Source: CAD feature listing. Evaluate the final solid. Frame: model axes, mm. Face numbers are marked on the shaded views. A direction names the side the tool comes from. Give positions to 0.01 mm unless a question says otherwise; leave off trailing zeros. Loops run counter-clockwise (first coordinate to the right, second up) from the corner with the lowest first, then second, coordinate; pieces in that order, holes last. Notation, with made-up numbers: M 23.5,26 L 32.5,26 A25 cw 32.5,50 Z; hole C 39,9 d7. An arc over 180 degrees is marked long. Put each result on its own line as item: value. Start each with the question number.
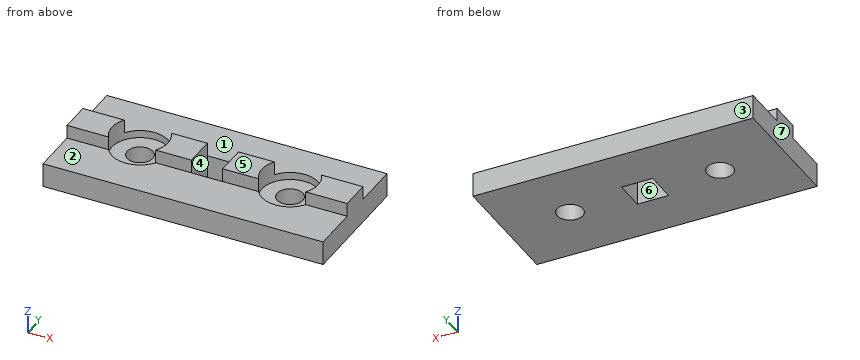
Autodesk Inventor part; units mm, degrees
ref_plane "i1_XY" through (-19.05, 0, -1.905) normal (0, 0, 1) x (1, 0, 0)
ref_plane "i1_YZ" through (-19.05, 0, -1.905) normal (1, 0, 0) x (0, 1, 0)
ref_plane "i1_ZX" through (-19.05, 0, -1.905) normal (0, 1, 0) x (0, 0, 1)
sketch "Sketch_1" plane through (0, 0, 0) normal (1, 0, 0) x (0, 1, 0)
  line L0 (3.9243, 3.429) -> (-3.9243, 3.429)
  line L1 (-3.9243, 3.429) -> (-3.9243, 0)
  line L2 (-3.9243, 0) -> (-15.875, 0)
  line L3 (-15.875, 0) -> (-15.875, -6.096)
  line L4 (-15.875, -6.096) -> (15.875, -6.096)
  line L5 (15.875, -6.096) -> (15.875, 0)
  line L6 (15.875, 0) -> (3.9243, 0)
  line L7 (3.9243, 0) -> (3.9243, 3.429)
extrude "Extrusion1" add sketch "Sketch_1" along normal mid plane 71.12
sketch "Sketch2" plane through (-35.56, 3.9243, 3.429) normal (0, 0, 1) x (1, 0, 0)
  point P0 (16.51, -3.9243)
hole "Drilling 1" at (-19.05, 0, 3.429) direction (0, 0, -1) diameter 6.5278 depth 9.525 counterbore diameter 14.2748 counterbore depth 5.334
sketch "Sketch3" plane through (35.56, -3.9243, 3.429) normal (0, 0, 1) x (1, 0, 0)
  point P0 (-16.51, 3.9243)
hole "Drilling 2" at (19.05, 0, 3.429) direction (0, 0, -1) diameter 6.5278 depth 9.525 counterbore diameter 14.2748 counterbore depth 5.334
sketch "Sketch_4" plane through (0, 0, 0) normal (0, 0, 1) x (1, 0, 0)
  line L0 (-3.9624, -3.9624) -> (3.9624, -3.9624)
  line L1 (3.9624, -3.9624) -> (3.9624, 3.9624)
  line L2 (3.9624, 3.9624) -> (-3.9624, 3.9624)
  line L3 (-3.9624, 3.9624) -> (-3.9624, -3.9624)
extrude "Extrusion2" cut sketch "Sketch_4" along normal mid plane 15.24
ref_plane "i1_XY" through (-19.05, 0, -1.905) normal (0, 0, 1) x (1, 0, 0)
ref_plane "i1_YZ" through (-19.05, 0, -1.905) normal (1, 0, 0) x (0, 1, 0)
ref_plane "i1_ZX" through (-19.05, 0, -1.905) normal (0, 1, 0) x (0, 0, 1)
ref_plane "i2_XY" through (19.05, 0, -1.905) normal (0, 0, 1) x (1, 0, 0)
ref_plane "i2_YZ" through (19.05, 0, -1.905) normal (1, 0, 0) x (0, 1, 0)
ref_plane "i2_ZX" through (19.05, 0, -1.905) normal (0, 1, 0) x (0, 0, 1)
ref_plane "pad_XY" through (-19.05, 0, -6.096) normal (0, 0, 1) x (1, 0, 0)
ref_plane "pad_YZ" through (-19.05, 0, -6.096) normal (1, 0, 0) x (0, 1, 0)
ref_plane "pad_ZX" through (-19.05, 0, -6.096) normal (0, 1, 0) x (0, 0, 1)
properties part number "6596_b"
1. Contact query for flat-ended pins moving along their axis: pin 1 (11.5 mm diameter, centred on x = -19.05, y = 0, fed in from +Z) (3 decimals); pin 2 (2.5 mm diameter, centred on x = 8, z = 2, fed in from -Y); pin 3 (2.5 mm diameter, centred on x = 10, z = 2, fed in from +Y). Output: stop coordinate, or through.
2. Section D-D, the plane z = -5. Output: boundary loops of the cut face in (x, y) (3 decimals).
3. Section C-C, the plane z = 1.5. Output: boundary loops of the cut face in (x, y).
4. Section B-B, the plane x = 2.5. Output: boundary loops of the cut face in (y, z) (3 decimals).
5. Set-up query: the marked faces 1, 2 and 3. Return all of +Z, -Z, +X, -X, +Y, -Y with unobstructed straight access to the full face (end or side cutting, diameter ignored); none if empty.
6. Ray query, line 1 (X direction, y = 0, z = -3.8); line 2 (X direction, y = 0, z = 1.5); line 3 (Y direction, x = -19.05, z = -4.25) (3 decimals). Return the intervals inside material, ascending.
7. Pull-direction query (X, two-part tool) for the marked faces 4, 5, 6 and 7; classes: released by +X, released by -X, zero draft, split by the parting line, or undercut.
8. Section A-A, the plane y = 0. Output: boundary loops of the cut face in (x, z) (3 decimals).
Results found:
1. pin 1: z = -1.905
1. pin 2: y = -3.92
1. pin 3: y = 3.92
2. outline: M -35.56,-15.875 L 35.56,-15.875 L 35.56,15.875 L -35.56,15.875 Z; hole C -19.05,0 d6.528; hole M -3.962,-3.962 L 3.962,-3.962 L 3.962,3.962 L -3.962,3.962 Z; hole C 19.05,0 d6.528
3. outline: M -35.56,-3.92 L -25.01,-3.92 A7.14 cw -25.01,3.92 L -35.56,3.92 Z; M -13.09,-3.92 L -3.96,-3.92 L -3.96,3.92 L -13.09,3.92 A7.14 cw Z; M 3.96,-3.92 L 13.09,-3.92 A7.14 cw 13.09,3.92 L 3.96,3.92 Z; M 25.01,-3.92 L 35.56,-3.92 L 35.56,3.92 L 25.01,3.92 A7.14 cw Z
4. outline: M -15.875,-6.096 L -3.962,-6.096 L -3.962,0 L -15.875,0 Z; M 3.962,-6.096 L 15.875,-6.096 L 15.875,0 L 3.962,0 Z
5. face 1: +Z, +X, -X, +Y
5. face 2: +Z, +X, -X, -Y
5. face 3: +Z, -Z, +X, -X, +Y
6. line 1: -35.56 to -22.31, -15.79 to -3.96, 3.96 to 15.79, 22.31 to 35.56
6. line 2: -35.56 to -26.19, -11.91 to -3.96, 3.96 to 11.91, 26.19 to 35.56
6. line 3: -15.875 to -3.264, 3.264 to 15.875
7. face 4: undercut
7. face 5: zero draft
7. face 6: undercut
7. face 7: released by -X
8. outline: M -35.56,-6.096 L -22.314,-6.096 L -22.314,-1.905 L -26.187,-1.905 L -26.187,3.429 L -35.56,3.429 Z; M -15.786,-6.096 L -3.962,-6.096 L -3.962,3.429 L -11.913,3.429 L -11.913,-1.905 L -15.786,-1.905 Z; M 3.962,-6.096 L 15.786,-6.096 L 15.786,-1.905 L 11.913,-1.905 L 11.913,3.429 L 3.962,3.429 Z; M 22.314,-6.096 L 35.56,-6.096 L 35.56,3.429 L 26.187,3.429 L 26.187,-1.905 L 22.314,-1.905 Z
